from build123d import *

# Parameters (mm, degrees)
SKETCH1_R           = 23.495
SKETCH1_R_2         = 3.81
SKETCH1_R_3         = 3.556
BOSS_EXTRUDE1_DEPTH = 3.175


with BuildPart() as part:
    # Sketch1 → Boss-Extrude1 (new body)
    with BuildSketch(Plane(origin=(0, 0, 0), x_dir=(1, 0, 0), z_dir=(0, 1, 0))):
        Circle(SKETCH1_R)
        with Locations((-11.055868466, 11.055868466)):
            Circle(SKETCH1_R_2, mode=Mode.SUBTRACT)
        Circle(SKETCH1_R_3, mode=Mode.SUBTRACT)
        with Locations((11.055868466, -11.055868466)):
            Circle(SKETCH1_R_2, mode=Mode.SUBTRACT)
        with Locations((11.055868466, 11.055868466)):
            Circle(SKETCH1_R_2, mode=Mode.SUBTRACT)
        with Locations((-11.055868466, -11.055868466)):
            Circle(SKETCH1_R_2, mode=Mode.SUBTRACT)
    extrude(amount=BOSS_EXTRUDE1_DEPTH)


solid = part.part
Read the model definition and answer for the solid it produces. Units are mm, in the model's axes. Give positions to 0.01 mm unless a question says otherwise; leave off trailing zeros. Write each loop counter-clockwise with the first axis right and the second up, starting at its lowest first coordinate (ties: lowest second). Pieces come first, ordered by that corner, then holes. Notation, with made-up numbers: (-21.5, 9) - (29.5, 9) arc R34 ccw to (29.5, 48) - close; hole circle Ø8 at (32, -9). An arc over 180 degrees is marked (long way). Use CSV: the item, a comma, the result in double quotes. Start each with the question number.
Item 1: The part is cut by section A-A, the plane z = 0. Give the vertices of the cut face in (x, y) (3 decimals).
Item 2: The part is cut by section C-C, the plane x = 12.5. Give the vertices of the cut face in (y, z) (3 decimals), and give its area (3 significant figures).
Item 3: Flat-ended cylindrical pins translate along their axes: P1, Ø1.5, axis at y = 2.5, z = -14.5, coming from the -X side; P2, Ø1, axis at x = -18, y = 1.5, coming from the -Z side. Find the tip coordinate at first contact, or state that the pin passes through.
Item 4: The part is cut by section B-B, the plane x = 0. Give the vertices of the cut face in (y, z) (3 decimals).
Item 5: Consider line 1 (X direction, y = 0.9, z = 10); line 2 (Z direction, x = -14.5, y = 2.4) (3 decimals); line 3 (Z direction, x = -9.5, y = 2.3). Determine where each line is inside the solid, lowest interval first.
Item 6: The part is cut by section D-D, the plane y = 2.2. Give the vertices of the cut face in (x, z) (3 decimals), and give its area (3 significant figures).
Item 7: The mould has two halves that part along Z. Classify faces 1 (the cylindrical face through (-7.422, 1.565, 9.911)), 2 (the cylindrical face through (-0.77, 1.57, 3.47)), 3 (the cylindrical face through (-5.093, 1.565, 22.936)), 4 (the flat face through (0, 3.175, 5)): pulls with the +Z half, pulls with the -Z half, needs draft (parallel to the pull), parting line crosses it, or undercut.
Taken from the geometry:
1,outline,"(-23.495, 0) - (-3.556, 0) - (-3.556, 3.175) - (-23.495, 3.175) - close; (3.556, 0) - (23.495, 0) - (23.495, 3.175) - (3.556, 3.175) - close"
2,outline,"(0, -19.894) - (3.175, -19.894) - (3.175, -14.582) - (0, -14.582) - close; (0, -7.53) - (3.175, -7.53) - (3.175, 7.53) - (0, 7.53) - close; (0, 14.582) - (3.175, 14.582) - (3.175, 19.894) - (0, 19.894) - close"
2,area,"81.5 mm2"
3,P1,"x = -19.05"
3,P2,"z = -15.68"
4,outline,"(0, -23.495) - (3.175, -23.495) - (3.175, -3.556) - (0, -3.556) - close; (0, 3.556) - (3.175, 3.556) - (3.175, 23.495) - (0, 23.495) - close"
5,line 1,"-21.26 to -14.72, -7.4 to 7.4, 14.72 to 21.26"
5,line 2,"-18.487 to -12.685, -9.427 to 9.427, 12.685 to 18.487"
5,line 3,"-21.49 to -14.53, -7.58 to 7.58, 14.53 to 21.49"
6,outline,"circle Ø46.99 at (0, 0); hole circle Ø7.62 at (-11.056, -11.056); hole circle Ø7.62 at (-11.056, 11.056); hole circle Ø7.112 at (0, 0); hole circle Ø7.62 at (11.056, -11.056); hole circle Ø7.62 at (11.056, 11.056)"
6,area,"1,510 mm2"
7,face 1,"undercut"
7,face 2,"undercut"
7,face 3,"parting line crosses it"
7,face 4,"needs draft"
